```python
from build123d import *

# Parameters (mm, degrees)
F0_W      = 70
F0_H      = 37.5
F0_W_2    = 90
F1_DEPTH  = 100
F2_DEPTH  = 80
F3_DEPTH  = 50
F0_W_3    = 180
F0_H_2    = 42
F4_DEPTH  = 40
F7_DEPTH  = 55
F8_DEPTH  = 4
F10_R     = 2
F11_W     = 154
F11_H     = 33.5
F11_W_2   = 117
F11_H_2   = 59
F11_W_3   = 172
F11_H_3   = 36
F12_DEPTH = 93


with BuildPart() as f1:
    # F0 (on Top) → F1 (new body)
    with BuildSketch(Plane.XY):
        with Locations((-35, 71.25)):
            Rectangle(F0_W, F0_H)
        with Locations((45, 71.25)):
            Rectangle(F0_W_2, F0_H)
        Polygon((-70, 52.5), (-70, 90), (-90, 90), (-90, 15), (-70, 15), align=None)
    extrude(amount=F1_DEPTH)

    # F0 (on Top) → F2 (join)
    with BuildSketch(Plane.XY):
        with Locations((-35, 33.75)):
            Rectangle(F0_W, F0_H)
        with Locations((45, 33.75)):
            Rectangle(F0_W_2, F0_H)
    extrude(amount=F2_DEPTH)

    # F0 (on Top) → F3 (join)
    with BuildSketch(Plane.XY):
        Polygon((90, -48), (90, 15), (0, 15), (-70, 15), (-90, 15), (-90, -48), align=None)
    extrude(amount=F3_DEPTH)

    # F0 (on Top) → F4 (join)
    with BuildSketch(Plane.XY):
        with Locations((0, -69)):
            Rectangle(F0_W_3, F0_H_2)
    extrude(amount=F4_DEPTH)

    # F6 (on face) → F7 (cut)
    with BuildSketch(Plane(origin=(-90, 0, 0), x_dir=(0, -1, 0), z_dir=(-1, 0, 0))):
        with BuildLine():
            ThreePointArc((-11.75, 50), (16.5, 21.75), (44.75, 50))
            Line((44.75, 50), (-11.75, 50))
        make_face()
    extrude(amount=-F7_DEPTH, mode=Mode.SUBTRACT)

    # F6 (on face) → F8 (join)
    with BuildSketch(Plane(origin=(-90, 0, 0), x_dir=(0, -1, 0), z_dir=(-1, 0, 0))):
        with BuildLine():
            ThreePointArc((-11.75, 50), (16.5, 21.75), (44.75, 50))
            Line((44.75, 50), (-11.75, 50))
        make_face()
    extrude(amount=-F8_DEPTH)

    # F10
    f10_edges = [f1.edges().sort_by_distance(p)[0] for p in [
        (-60.5, 11.75, 50),
        (-35, -16.5, 50),
        (-60.5, -44.75, 50),
        (-86, -16.5, 50),
    ]]
    fillet(f10_edges, radius=F10_R)

    # F11 (on offset) → F12 (cut)
    with BuildSketch(Plane.XY.offset(100)):
        Polygon((-86, 17), (-72, 17), (-72, 52.5), (-72, 54.5), (-70, 54.5), (86, 54.5), (86, 86), (-86, 86), align=None)
        with Locations((9, 33.75)):
            Rectangle(F11_W, F11_H)
        with Locations((27.5, -16.5)):
            Rectangle(F11_W_2, F11_H_2)
        with Locations((0, -68)):
            Rectangle(F11_W_3, F11_H_3)
    extrude(amount=-F12_DEPTH, mode=Mode.SUBTRACT)


solid = f1.part
```
Verification items for the finished model (mm, model axes). A direction names the side the tool comes from. Give positions to 0.01 mm unless a question says otherwise; leave off trailing zeros. Loops run counter-clockwise (first coordinate to the right, second up) from the corner with the lowest first, then second, coordinate; pieces in that order, holes last. Notation, with made-up numbers: M 66.5,12 L 120.5,12 A13 ccw 120.5,19 Z; hole C 28,26.5 d2. An arc over 180 degrees is marked long. One line per question, with ' | ' between items.
Item 1: Section check C-C, the plane x = 41.5. Record the cut outline in (y, z).
Completed:
outline: M -90,0 L 90,0 L 90,100 L 86,100 L 86,7 L 54.5,7 L 54.5,100 L 52.5,100 L 52.5,80 L 50.5,80 L 50.5,7 L 17,7 L 17,80 L 15,80 L 15,50 L 13,50 L 13,7 L -46,7 L -46,50 L -48,50 L -48,40 L -50,40 L -50,7 L -86,7 L -86,40 L -90,40 Z
Item 2: Section check D-D, the plane z = 68. Record the cut outline in (x, y), plus the area to 3 significant figures.
Completed:
outline: M -90,15 L 90,15 L 90,90 L -90,90 Z; hole M -86,17 L -72,17 L -72,54.5 L 86,54.5 L 86,86 L -86,86 Z; hole M -68,17 L 86,17 L 86,50.5 L -68,50.5 Z | area: 2,400 mm^2
Item 3: Draft check along Y on faces 3 (the face through (86, -17, 29)), 4 (the face through (1, 90, 49)), 5 (the face through (0, -89, 40)). Enter one of: +Y half, -Y half, draft (parallel to the pull), parting line (faces both ways), or undercut.
Completed:
face 3: undercut | face 4: +Y half | face 5: draft
Item 4: Section check A-A, the plane z = 89. Record the cut outline in (x, y).
Completed:
outline: M -90,15 L -70,15 L -70,52.5 L 90,52.5 L 90,90 L -90,90 Z; hole M -86,17 L -72,17 L -72,54.5 L 86,54.5 L 86,86 L -86,86 Z
Item 5: Depth check by flat-ended pin: P1, Ø1.5, axis at x = -21, z = 44.5, coming from the -Y side; P2, Ø16, axis at y = 28.5, z = 93.5, coming from the +X side; P3, Ø8, axis at x = 46.5, y = 13.5, coming from the +Z side. Enter the tip coordinate at first touch or a pass-through.
Completed:
P1: stops at y = -48 | P2: stops at x = -70 | P3: stops at z = 80
Item 6: Thickness scan on line 1 (X direction, y = 17.5, z = 79.5); line 2 (Y direction, x = -47, z = 79.5); line 3 (Y direction, x = -13.5, z = 18). Record the ranges inside material, lowest first. Write a range as [from, to].
Completed:
line 1: x = [-90, -86], [-72, -68], [86, 90] | line 2: y = [15, 17], [50.5, 54.5], [86, 90] | line 3: y = [-90, -86], [-50, -46], [13, 17], [50.5, 54.5], [86, 90]
Item 7: Section check B-B, the plane y = 33. Record the cut outline in (x, z), plus the area to 3 significant figures.
Completed:
outline: M -90,0 L 90,0 L 90,80 L 86,80 L 86,7 L -68,7 L -68,80 L -70,80 L -70,100 L -72,100 L -72,7 L -86,7 L -86,100 L -90,100 Z | area: 2,260 mm^2
Item 8: Tool access check on faces 1 (the face through (86, 34, 44)), 2 (the face through (-90, 21, 40)). Record the directions out of +Z, -Z, +X, -X, +Y, -Y that give a thin tool (end or side, any length) a straight path to the whole face; none if there is none.
Completed:
face 1: +Z | face 2: +Z, -Z, -X, +Y, -Y
